For this review, take the finished solid that the model builds, in its own axes (mm). A direction names the side the tool comes from. Round coordinates to 2 decimals unless told otherwise and drop trailing zeros. Order: outer loops, then holes, each group sorted by start corner. A loop starts at its lowest first (then second) coordinate and runs counter-clockwise, first axis right, second up. Notation, with made-up numbers: (-14.75, -10) -> (37.25, -10) arc R13 ccw to (37.25, 0) -> close; hole circle Ø5 at (22, 62.25). An arc over 180 degrees is marked (long way). Put each result on its own line as item: value. Start each with the question number.
```python
from build123d import *

# Parameters (mm, degrees)
SKETCH1_W           = 36
SKETCH1_H           = 81
BOSS_EXTRUDE1_DEPTH = 11
SKETCH2_W           = 30
SKETCH2_H           = 75
CUT_EXTRUDE1_DEPTH  = 8
FILLET1_R           = 3
SKETCH3_W           = 1.6
SKETCH3_H           = 3
CUT_EXTRUDE2_DEPTH  = 0.8
SKETCH4_W           = 1
SKETCH4_H           = 5
SKETCH4_W_2         = 5
SKETCH4_H_2         = 1
BOSS_EXTRUDE2_DEPTH = 2
SKETCH5_W           = 8.5
SKETCH5_H           = 14
SKETCH5_W_2         = 15
SKETCH5_H_2         = 27
CUT_EXTRUDE4_DEPTH  = 8


with BuildPart() as part:
    # Sketch1 → Boss-Extrude1 (new body)
    with BuildSketch(Plane(origin=(0, 0, 0), x_dir=(1, 0, 0), z_dir=(0, 1, 0))):
        with Locations((18, 40.5)):
            Rectangle(SKETCH1_W, SKETCH1_H)
    extrude(amount=BOSS_EXTRUDE1_DEPTH)

    # Sketch2 → Cut-Extrude1 (cut)
    with BuildSketch(Plane(origin=(0, 11, 0), x_dir=(1, 0, 0), z_dir=(0, 1, 0))):
        with Locations((18, 40.5)):
            Rectangle(SKETCH2_W, SKETCH2_H)
    extrude(amount=-CUT_EXTRUDE1_DEPTH, mode=Mode.SUBTRACT)

    # Fillet1
    fillet1_edges = [part.edges().sort_by_distance(p)[0] for p in [
        (0, 5.5, -81),
        (36, 5.5, -81),
        (36, 5.5, 0),
        (0, 5.5, 0),
    ]]
    fillet(fillet1_edges, radius=FILLET1_R)

    # Sketch3 → Cut-Extrude2 (cut)
    with BuildSketch(Plane(origin=(0, 11, 0), x_dir=(1, 0, 0), z_dir=(0, 1, 0))):
        with Locations((18, 79.5)):
            Rectangle(SKETCH3_W, SKETCH3_H)
    extrude(amount=-CUT_EXTRUDE2_DEPTH, mode=Mode.SUBTRACT)

    # Sketch4 → Boss-Extrude2 (add)
    with BuildSketch(Plane(origin=(0, 11, 0), x_dir=(1, 0, 0), z_dir=(0, 1, 0))):
        with Locations((2.5, 40.5)):
            Rectangle(SKETCH4_W, SKETCH4_H)
        with Locations((33.5, 40.5)):
            Rectangle(SKETCH4_W, SKETCH4_H)
        with Locations((18, 2.5)):
            Rectangle(SKETCH4_W_2, SKETCH4_H_2)
    extrude(amount=BOSS_EXTRUDE2_DEPTH)

    # Sketch5 → Cut-Extrude4 (cut)
    with BuildSketch(Plane.XZ):
        with Locations((7.25, -71)):
            Rectangle(SKETCH5_W, SKETCH5_H)
        with Locations((20.5, -37.5)):
            Rectangle(SKETCH5_W_2, SKETCH5_H_2)
    extrude(amount=-CUT_EXTRUDE4_DEPTH, mode=Mode.SUBTRACT)


solid = part.part
```
Item 1: Consider section B-B, the plane y = 8.75. Write out the cut boundary in (x, z), plus the area to 3 significant figures.
Item 2: Consider section A-A, the plane z = -66. Write out the cut boundary in (x, y), plus the area to 4 significant figures.
Item 3: For L1, parallel to X at y = 10.75, z = -52.5; L2, parallel to Z at x = 12.5, y = 8.25; L3, parallel to Y at x = 31.5, z = -47, list the stretches that pass through material, from the lowest coordinate up.
Item 4: Consider section D-D, the plane z = -36.5. Write out the cut boundary in (x, y).
Item 5: Mouldability with a two-part tool opening along Z and no side actions: class faces 1 (the face through (20, 1, -24)), 2 (the face through (35.1, 5.58, -80.14)), 3 (the face through (2, 12, -40)) as +Z half, -Z half, draft (parallel to the pull), parting line (faces both ways), or undercut.
Item 6: Tool access review of faces 4 (the face through (18, 7, -78)), 5 (the face through (18, 10.2, -80)), 6 (the face through (34, 12, -40)), 7 (the face through (18, 12, -2)): name each direction out of +Z, -Z, +X, -X, +Y, -Y from which nothing blocks a thin tool from reaching the whole face with its end or side.
Item 7: Insertion check: pin 1 Ø0.5 at (x, y) = (2.5, 12) entering from -Z; pin 2 Ø0.8 at (x, y) = (2.5, 12) entering from +Z; pin 3 Ø1 at (y, z) = (12, -41.5) entering from +X. Each pin has a flat end and moves straight along its axis. Give the tip position at first contact, or say it passes through.
Item 8: Consider section C-C, the plane x = 22. Write out the cut boundary in (y, z).
Evaluation:
1. outline: (0, -78) arc R3 ccw to (3, -81) -> (33, -81) arc R3 ccw to (36, -78) -> (36, -3) arc R3 ccw to (33, 0) -> (3, 0) arc R3 ccw to (0, -3) -> close; hole (3, -78) -> (33, -78) -> (33, -3) -> (3, -3) -> close
1. area: 658 mm^2
2. outline: (0, 0) -> (3, 0) -> (3, 11) -> (0, 11) -> close; (11.5, 0) -> (36, 0) -> (36, 11) -> (33, 11) -> (33, 3) -> (11.5, 3) -> close
2. area: 130.5 mm^2
3. L1: x = 0 to 3, 33 to 36
3. L2: z = -81 to -78, -3 to 0
3. L3: y = 0 to 3
4. outline: (0, 0) -> (13, 0) -> (13, 3) -> (3, 3) -> (3, 11) -> (0, 11) -> close; (28, 0) -> (36, 0) -> (36, 11) -> (33, 11) -> (33, 3) -> (28, 3) -> close
5. face 1: undercut
5. face 2: -Z half
5. face 3: draft
6. face 4: +Y
6. face 5: -Z, +Y
6. face 6: +Z, -Z, +X, +Y
6. face 7: +Z, +X, -X, +Y
7. pin 1: stops at z = -43
7. pin 2: stops at z = -38
7. pin 3: stops at x = 34
8. outline: (0, -81) -> (11, -81) -> (11, -78) -> (3, -78) -> (3, -51) -> (0, -51) -> close; (0, -24) -> (3, -24) -> (3, -3) -> (11, -3) -> (11, 0) -> (0, 0) -> close
